Study the drawing (mm; zero at the part's minimum x, y, z) and answer. A direction names the side the tool comes from. Coordinates: 2 decimals unless noted, no trailing zeros. Write each loop counter-clockwise with the first axis right and the second up, starting at its lowest first coordinate (ties: lowest second). Pieces come first, ordered by that corner, then holes. Notation, with made-up numbers: M 1.5,11 L 50.5,11 A31 ccw 50.5,39 Z; hole C -2.75,74 d10. An arc over 180 degrees is marked long. Answer as a JSON object with one key per item and string values. Group by question number.
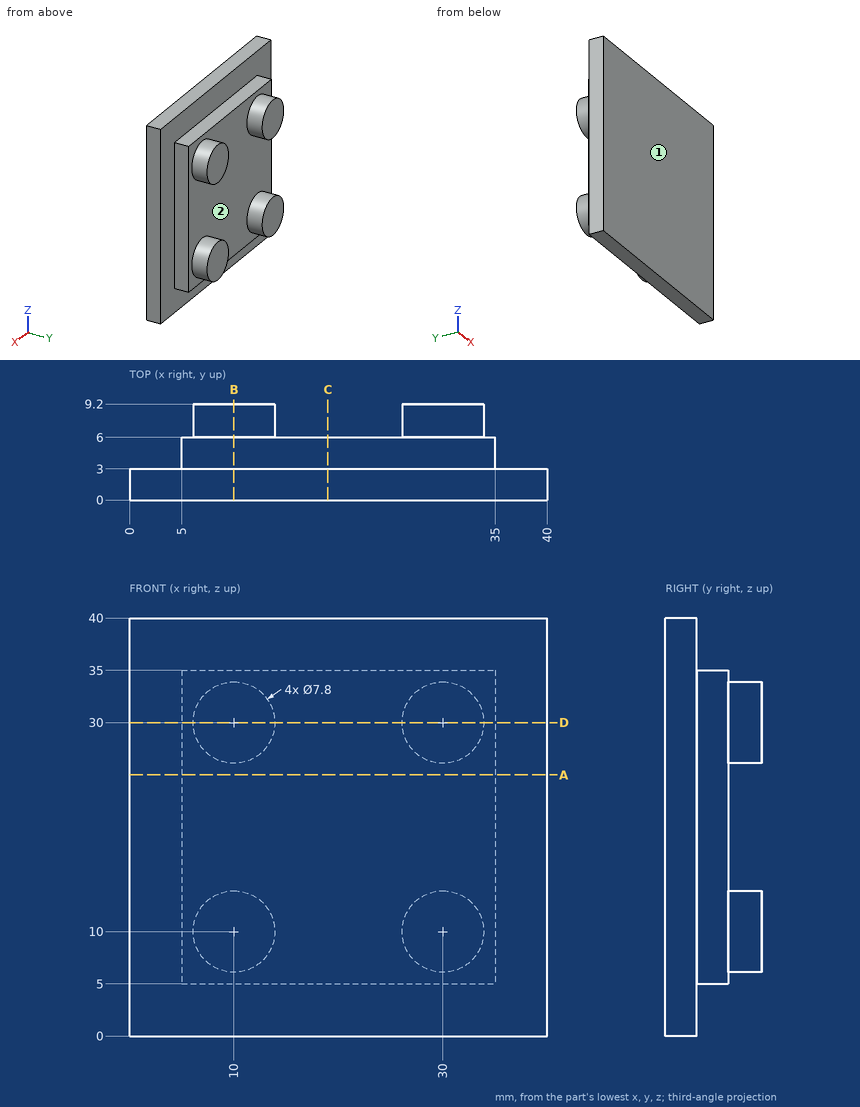
Item 1: Flat-ended cylindrical pins translate along their axes: pin 1 Ø0.9 at (x, y) = (25.5, 5) entering from +Z; pin 2 Ø2.5 at (x, y) = (20, 5) entering from -Z; pin 3 Ø10 at (x, z) = (20.5, 13) entering from +Y; pin 4 Ø24 at (x, z) = (24, 18.5) entering from +Y. Find the tip coordinate at first contact, or state that the pin passes through.
Item 2: A cutting plane is placed at D-D, the plane z = 30. Write down the section's boundary in (x, y), and give its area (3 significant figures).
Item 3: A tool of negligible diameter and unlimited length cuts with its end or side. For the marked faces 1 and 2, from which of +Z, -Z, +X, -X, +Y, -Y can it reach the whole face along a straight path? Write none if from no direction.
Item 4: A cutting plane is placed at B-B, the plane x = 10. Write down the section's boundary in (y, z), and give its area (3 significant figures).
Item 5: A cutting plane is placed at C-C, the plane x = 19. Write down the section's boundary in (y, z), and give its area (3 significant figures).
Item 6: A cutting plane is placed at A-A, the plane z = 25. Write down the section's boundary in (x, y), and give its area (3 significant figures).
Item 7: Consider L1, parallel to X at y = 7, z = 30; L2, parallel to Y at x = 13, z = 36.5; L3, parallel to X at y = 4.5, z = 14.5. Determine where each line is inside the solid, lowest interval first. Write a range as from..to.
Answer:
{
 "1": {"pin 1": "z = 35", "pin 2": "z = 5", "pin 3": "y = 6", "pin 4": "y = 9.2"},
 "2": {"outline": "M 0,0 L 40,0 L 40,3 L 35,3 L 35,6 L 33.9,6 L 33.9,9.2 L 26.1,9.2 L 26.1,6 L 13.9,6 L 13.9,9.2 L 6.1,9.2 L 6.1,6 L 5,6 L 5,3 L 0,3 Z", "area": "260 mm2"},
 "3": {"face 1": "+Z, -Z, +X, -X, -Y", "face 2": "+Y"},
 "4": {"outline": "M 0,0 L 3,0 L 3,5 L 6,5 L 6,6.1 L 9.2,6.1 L 9.2,13.9 L 6,13.9 L 6,26.1 L 9.2,26.1 L 9.2,33.9 L 6,33.9 L 6,35 L 3,35 L 3,40 L 0,40 Z", "area": "260 mm2"},
 "5": {"outline": "M 0,0 L 3,0 L 3,5 L 6,5 L 6,35 L 3,35 L 3,40 L 0,40 Z", "area": "210 mm2"},
 "6": {"outline": "M 0,0 L 40,0 L 40,3 L 35,3 L 35,6 L 5,6 L 5,3 L 0,3 Z", "area": "210 mm2"},
 "7": {"L1": "6.1..13.9, 26.1..33.9", "L2": "0..3", "L3": "5..35"}
}
